Here's how the part is built. I have some questions about the finished solid (model axes, mm). Coordinates: 2 decimals unless noted, no trailing zeros. Write each loop counter-clockwise with the first axis right and the second up, starting at its lowest first coordinate (ties: lowest second). Pieces come first, ordered by that corner, then holes.
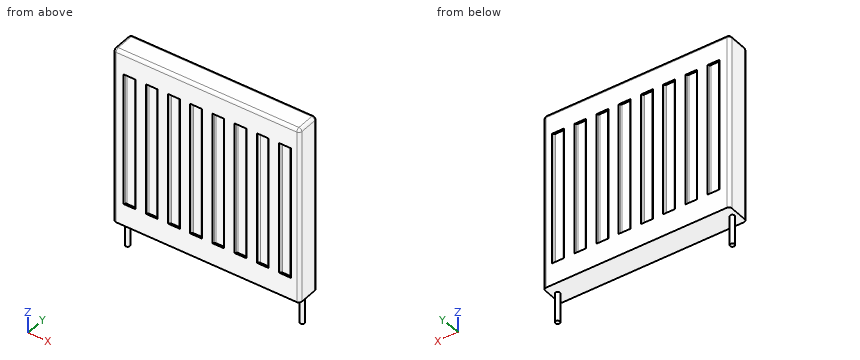
```python
from build123d import *

# Parameters (mm, degrees)
F0_W     = 630
F0_H     = 80
F1_DEPTH = 300
F2_R     = 7.5
F3_DEPTH = 100
F5_DEPTH = 225
F6_R     = 10


with BuildPart() as f1:
    # F0 (on Top) → F1 (new body, symmetric)
    with BuildSketch(Plane.XY):
        with Locations((-30.66069, -58.683639)):
            Rectangle(F0_W, F0_H)
    extrude(amount=F1_DEPTH, both=True)

    # F2 (on face) → F3 (join)
    with BuildSketch(Plane(origin=(0, 0, -300), x_dir=(1, 0, 0), z_dir=(0, 0, -1))):
        with Locations((264.33931, 58.683639)):
            Circle(F2_R)
        with Locations((-325.66069, 58.683639)):
            Circle(F2_R)
    extrude(amount=F3_DEPTH)

    # F4 (on Top) → F5 (cut, symmetric)
    with BuildSketch(Plane.XY):
        with BuildLine():
            Line((-270.66069, -18.683639), (-310.66069, -18.683639))
            Line((-310.66069, -18.683639), (-307.124776, -22.897577))
            ThreePointArc((-307.124776, -22.897577), (-305.407645, -24.215178), (-303.294554, -24.683639))
            Line((-303.294554, -24.683639), (-278.026826, -24.683639))
            ThreePointArc((-278.026826, -24.683639), (-275.913735, -24.215178), (-274.196604, -22.897577))
            Line((-274.196604, -22.897577), (-270.66069, -18.683639))
        make_face()
        with BuildLine():
            Line((-195.66069, -18.683639), (-235.66069, -18.683639))
            Line((-235.66069, -18.683639), (-232.124776, -22.897577))
            ThreePointArc((-232.124776, -22.897577), (-230.407645, -24.215178), (-228.294554, -24.683639))
            Line((-228.294554, -24.683639), (-203.026826, -24.683639))
            ThreePointArc((-203.026826, -24.683639), (-200.913735, -24.215178), (-199.196604, -22.897577))
            Line((-199.196604, -22.897577), (-195.66069, -18.683639))
        make_face()
        with BuildLine():
            Line((-120.66069, -18.683639), (-160.66069, -18.683639))
            Line((-160.66069, -18.683639), (-157.124776, -22.897577))
            ThreePointArc((-157.124776, -22.897577), (-155.407645, -24.215178), (-153.294554, -24.683639))
            Line((-153.294554, -24.683639), (-128.026826, -24.683639))
            ThreePointArc((-128.026826, -24.683639), (-125.913735, -24.215178), (-124.196604, -22.897577))
            Line((-124.196604, -22.897577), (-120.66069, -18.683639))
        make_face()
        with BuildLine():
            Line((-45.66069, -18.683639), (-85.66069, -18.683639))
            Line((-85.66069, -18.683639), (-82.124776, -22.897577))
            ThreePointArc((-82.124776, -22.897577), (-80.407645, -24.215178), (-78.294554, -24.683639))
            Line((-78.294554, -24.683639), (-53.026826, -24.683639))
            ThreePointArc((-53.026826, -24.683639), (-50.913735, -24.215178), (-49.196604, -22.897577))
            Line((-49.196604, -22.897577), (-45.66069, -18.683639))
        make_face()
        with BuildLine():
            Line((29.33931, -18.683639), (-10.66069, -18.683639))
            Line((-10.66069, -18.683639), (-7.124776, -22.897577))
            ThreePointArc((-7.124776, -22.897577), (-5.407645, -24.215178), (-3.294554, -24.683639))
            Line((-3.294554, -24.683639), (21.973174, -24.683639))
            ThreePointArc((21.973174, -24.683639), (24.086265, -24.215178), (25.803396, -22.897577))
            Line((25.803396, -22.897577), (29.33931, -18.683639))
        make_face()
        with BuildLine():
            Line((104.33931, -18.683639), (64.33931, -18.683639))
            Line((64.33931, -18.683639), (67.875224, -22.897577))
            ThreePointArc((67.875224, -22.897577), (69.592355, -24.215178), (71.705446, -24.683639))
            Line((71.705446, -24.683639), (96.973174, -24.683639))
            ThreePointArc((96.973174, -24.683639), (99.086265, -24.215178), (100.803396, -22.897577))
            Line((100.803396, -22.897577), (104.33931, -18.683639))
        make_face()
        with BuildLine():
            Line((179.33931, -18.683639), (139.33931, -18.683639))
            Line((139.33931, -18.683639), (142.875224, -22.897577))
            ThreePointArc((142.875224, -22.897577), (144.592355, -24.215178), (146.705446, -24.683639))
            Line((146.705446, -24.683639), (171.973174, -24.683639))
            ThreePointArc((171.973174, -24.683639), (174.086265, -24.215178), (175.803396, -22.897577))
            Line((175.803396, -22.897577), (179.33931, -18.683639))
        make_face()
        with BuildLine():
            Line((254.33931, -18.683639), (214.33931, -18.683639))
            Line((214.33931, -18.683639), (217.875224, -22.897577))
            ThreePointArc((217.875224, -22.897577), (219.592355, -24.215178), (221.705446, -24.683639))
            Line((221.705446, -24.683639), (246.973174, -24.683639))
            ThreePointArc((246.973174, -24.683639), (249.086265, -24.215178), (250.803396, -22.897577))
            Line((250.803396, -22.897577), (254.33931, -18.683639))
        make_face()
        with BuildLine():
            ThreePointArc((-303.294554, -92.683639), (-305.407645, -93.1521), (-307.124776, -94.469701))
            Line((-307.124776, -94.469701), (-310.66069, -98.683639))
            Line((-310.66069, -98.683639), (-270.66069, -98.683639))
            Line((-270.66069, -98.683639), (-274.196604, -94.469701))
            ThreePointArc((-274.196604, -94.469701), (-275.913735, -93.1521), (-278.026826, -92.683639))
            Line((-278.026826, -92.683639), (-303.294554, -92.683639))
        make_face()
        with BuildLine():
            Line((-232.124776, -94.469701), (-235.66069, -98.683639))
            Line((-235.66069, -98.683639), (-195.66069, -98.683639))
            Line((-195.66069, -98.683639), (-199.196604, -94.469701))
            ThreePointArc((-199.196604, -94.469701), (-200.913735, -93.1521), (-203.026826, -92.683639))
            Line((-203.026826, -92.683639), (-228.294554, -92.683639))
            ThreePointArc((-228.294554, -92.683639), (-230.407645, -93.1521), (-232.124776, -94.469701))
        make_face()
        with BuildLine():
            ThreePointArc((250.803396, -94.469701), (249.086265, -93.1521), (246.973174, -92.683639))
            Line((246.973174, -92.683639), (221.705446, -92.683639))
            ThreePointArc((221.705446, -92.683639), (219.592355, -93.1521), (217.875224, -94.469701))
            Line((217.875224, -94.469701), (214.33931, -98.683639))
            Line((214.33931, -98.683639), (254.33931, -98.683639))
            Line((254.33931, -98.683639), (250.803396, -94.469701))
        make_face()
        with BuildLine():
            Line((-82.124776, -94.469701), (-85.66069, -98.683639))
            Line((-85.66069, -98.683639), (-45.66069, -98.683639))
            Line((-45.66069, -98.683639), (-49.196604, -94.469701))
            ThreePointArc((-49.196604, -94.469701), (-50.913735, -93.1521), (-53.026826, -92.683639))
            Line((-53.026826, -92.683639), (-78.294554, -92.683639))
            ThreePointArc((-78.294554, -92.683639), (-80.407645, -93.1521), (-82.124776, -94.469701))
        make_face()
        with BuildLine():
            Line((-120.66069, -98.683639), (-124.196604, -94.469701))
            ThreePointArc((-124.196604, -94.469701), (-125.913735, -93.1521), (-128.026826, -92.683639))
            Line((-128.026826, -92.683639), (-153.294554, -92.683639))
            ThreePointArc((-153.294554, -92.683639), (-155.407645, -93.1521), (-157.124776, -94.469701))
            Line((-157.124776, -94.469701), (-160.66069, -98.683639))
            Line((-160.66069, -98.683639), (-120.66069, -98.683639))
        make_face()
        with BuildLine():
            Line((-7.124776, -94.469701), (-10.66069, -98.683639))
            Line((-10.66069, -98.683639), (29.33931, -98.683639))
            Line((29.33931, -98.683639), (25.803396, -94.469701))
            ThreePointArc((25.803396, -94.469701), (24.086265, -93.1521), (21.973174, -92.683639))
            Line((21.973174, -92.683639), (-3.294554, -92.683639))
            ThreePointArc((-3.294554, -92.683639), (-5.407645, -93.1521), (-7.124776, -94.469701))
        make_face()
        with BuildLine():
            Line((104.33931, -98.683639), (100.803396, -94.469701))
            ThreePointArc((100.803396, -94.469701), (99.086265, -93.1521), (96.973174, -92.683639))
            Line((96.973174, -92.683639), (71.705446, -92.683639))
            ThreePointArc((71.705446, -92.683639), (69.592355, -93.1521), (67.875224, -94.469701))
            Line((67.875224, -94.469701), (64.33931, -98.683639))
            Line((64.33931, -98.683639), (104.33931, -98.683639))
        make_face()
        with BuildLine():
            Line((142.875224, -94.469701), (139.33931, -98.683639))
            Line((139.33931, -98.683639), (179.33931, -98.683639))
            Line((179.33931, -98.683639), (175.803396, -94.469701))
            ThreePointArc((175.803396, -94.469701), (174.086265, -93.1521), (171.973174, -92.683639))
            Line((171.973174, -92.683639), (146.705446, -92.683639))
            ThreePointArc((146.705446, -92.683639), (144.592355, -93.1521), (142.875224, -94.469701))
        make_face()
    extrude(amount=F5_DEPTH, both=True, mode=Mode.SUBTRACT)

    # F6
    f6_edges = [f1.edges().sort_by_distance(p)[0] for p in [
        (-345.66069, -98.683639, 0),
        (-345.66069, -18.683639, 0),
        (284.33931, -98.683639, 0),
        (284.33931, -18.683639, 0),
        (-30.66069, -98.683639, 300),
        (-30.66069, -18.683639, 300),
        (284.33931, -58.683639, 300),
        (-345.66069, -58.683639, 300),
    ]]
    fillet(f6_edges, radius=F6_R)


solid = f1.part
```
1) Will these pins go through, and if not, where does the flat tip stop? pin 1 (20 mm diameter, centred on x = 236.5, z = -100.5, fed in from -Y); pin 2 (5 mm diameter, centred on x = -221, y = -95.5, fed in from -Z); pin 3 (6.5 mm diameter, centred on x = 242, y = -96, fed in from +Z).
Values follow:
pin 1: stops at y = -92.68
pin 2: stops at z = -300
pin 3: stops at z = 299.14
2) I need wall thicknesses on probe 1 along Y at (x, z) = (8.5, -28.5); probe 2 along Z at (x, y) = (-94.5, -37.5); probe 3 along X at (y, z) = (-61, -349.5). Which ranges of each line are inside material? Lowest first, please.
Values follow:
probe 1: y = -92.68 to -24.68
probe 2: z = -300 to 300
probe 3: x = -332.79 to -318.53, 257.21 to 271.47
3) Imagine slicing it at A-A on x = -26. Please give me the cut outline in (y, z).
Values follow:
outline: (-98.68, -300) - (-18.68, -300) - (-18.68, 290) arc R10 ccw to (-28.68, 300) - (-88.68, 300) arc R10 ccw to (-98.68, 290) - close
4) Imagine slicing it at C-C on z = -330. Please give me the cut outline in (x, y).
Values follow:
outline: circle Ø15 at (-325.66, -58.68); circle Ø15 at (264.34, -58.68)
5) Imagine slicing it at B-B on y = -75. Please give me the cut outline in (x, z), then the cut area to 3 significant figures.
Values follow:
outline: (-345.66, -300) - (284.34, -300) - (284.34, 290) arc R10 ccw to (274.34, 300) - (-335.66, 300) arc R10 ccw to (-345.66, 290) - close
area: 378,000 mm2
